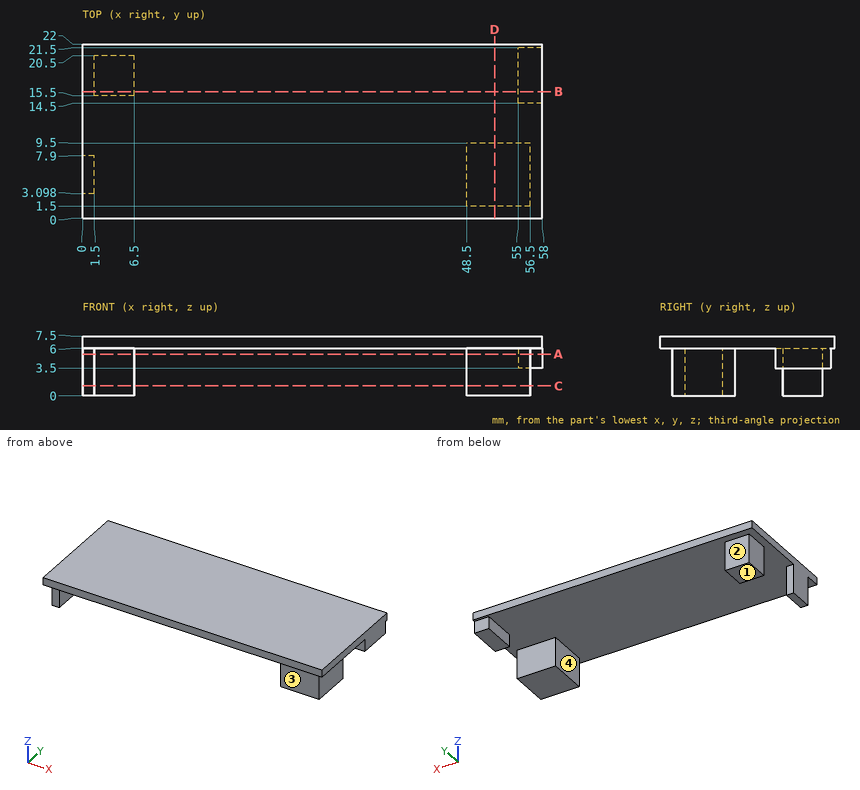
The drawing under review shows one solid part. Ordinate dimensions are in mm from its lowest x, y, z. A direction names the side the tool comes from. Coordinates: 2 decimals unless noted, no trailing zeros. Write each loop counter-clockwise with the first axis right and the second up, starting at its lowest first coordinate (ties: lowest second). Pieces come first, ordered by that corner, then holes.
1) To check wall thickness, follow L1, parallel to X at y = 7.5, z = 2.5; L2, parallel to Z at x = 25.5, y = 20.5; L3, parallel to X at y = 16.5, z = 3.25. State the ranges of each line that lie inside material, in increasing order.
2) Machinability: for the marked faces 1 and 2, which of the approach directions +Z, -Z, +X, -X, +Y, -Y give a long, thin tool a straight path to every point of the face, cutting with its end or side? Answer none if there is none.
3) Mouldability with a two-part tool opening along X and no side actions: class the marked faces 3 and 4 as +X half, -X half, draft (parallel to the pull), parting line (faces both ways), or undercut.
4) Add section B-B (y = 16). Write out the cut boundary in (x, z), plus the area to 4 significant figures.
5) Add section A-A (z = 5.25). Write out the cut boundary in (x, y), plus the area to 3 significant figures.
6) Insertion check: pin 1 (2 mm diameter, centred on x = 56, z = 4.5, fed in from +Y); pin 2 (1.2 mm diameter, centred on x = 1, z = 3, fed in from -Y); pin 3 (2.5 mm diameter, centred on x = 4.5, z = 4, fed in from -Y); pin 4 (1.5 mm diameter, centred on y = 2.5, z = 3, fed in from -X). Each pin has a flat end and moves straight along its axis. Give the tip position at first contact, or say it passes through.
7) Add section C-C (z = 1.25). Write out the cut boundary in (x, y), plus the area to 3 significant figures.
8) Add section D-D (x = 52). Write out the cut boundary in (y, z).
Check result:
1. L1: x = 0 to 1.5, 48.5 to 56.5
1. L2: z = 6 to 7.5
1. L3: x = 1.5 to 6.5
2. face 1: -Z, +X, -X, +Y, -Y
2. face 2: -Z, -X, +Y
3. face 3: draft
3. face 4: undercut
4. outline: (0, 6) - (1.5, 6) - (1.5, 0) - (6.5, 0) - (6.5, 6) - (55, 6) - (55, 3.5) - (58, 3.5) - (58, 7.5) - (0, 7.5) - close
4. area: 124.5 mm2
5. outline: (0, 3.1) - (1.5, 3.1) - (1.5, 7.9) - (0, 7.9) - close; (1.5, 15.5) - (6.5, 15.5) - (6.5, 20.5) - (1.5, 20.5) - close; (48.5, 1.5) - (56.5, 1.5) - (56.5, 9.5) - (48.5, 9.5) - close; (55, 14.5) - (58, 14.5) - (58, 21.5) - (55, 21.5) - close
5. area: 117 mm2
6. pin 1: stops at y = 21.5
6. pin 2: stops at y = 3.1
6. pin 3: stops at y = 15.5
6. pin 4: stops at x = 0
7. outline: (0, 3.1) - (1.5, 3.1) - (1.5, 7.9) - (0, 7.9) - close; (1.5, 15.5) - (6.5, 15.5) - (6.5, 20.5) - (1.5, 20.5) - close; (48.5, 1.5) - (56.5, 1.5) - (56.5, 9.5) - (48.5, 9.5) - close
7. area: 96.2 mm2
8. outline: (0, 6) - (1.5, 6) - (1.5, 0) - (9.5, 0) - (9.5, 6) - (22, 6) - (22, 7.5) - (0, 7.5) - close
